Check sheet for the modelled part. Datum: model origin and axes. Units: mm. A direction names the side the tool comes from. Coordinates: 2 decimals unless noted, no trailing zeros. Order: outer loops, then holes, each group sorted by start corner. A loop starts at its lowest first (then second) coordinate and runs counter-clockwise, first axis right, second up. Notation, with made-up numbers: (52.5, -21) -> (101.5, -21) arc R24 cw to (101.5, -10) -> close; hole circle Ø1 at (-15, -3.75). An arc over 180 degrees is marked (long way). Put each result on its own line as item: value. Start each with the question number.
```python
from build123d import *

# Parameters (mm, degrees)
F0_W     = 309.716136
F0_H     = 25.80601
F1_DEPTH = 114.3
F2_T     = -2.54


with BuildPart() as f1:
    # F0 (on Right) → F1 (new body)
    with BuildSketch(Plane.YZ):
        Rectangle(F0_W, F0_H)
    extrude(amount=F1_DEPTH)

    # F2
    f2_openings = [f1.faces().sort_by_distance(p)[0] for p in [
        (57.15, -154.858068, 0),
        (57.15, 0, 12.903005),
        (114.3, 0, 0),
        (57.15, 154.858068, 0),
    ]]
    offset(amount=F2_T, openings=f2_openings)


solid = f1.part
```
1) Gauge pin test, flat ends, axial feed: pin 1 (2 mm diameter, centred on y = 106, z = 4.5, fed in from +X); pin 2 (3 mm diameter, centred on x = 15, y = -82.5, fed in from +Z). Record the tip position at first contact, or that the pin passes through.
2) Sectioned sample at A-A (y = -115.5). Record the boundary of the cut face in (x, z).
3) Scan lines: line 1 along X through (y, z) = (-29, 10); line 2 along Z through (x, y) = (103, -69). Record each from-to range of solid material in increasing order. Write a range as [from, to].
4) Access from +Z, -Z, +X, -X, +Y, -Y to the whole of each face (thin tool, end or side, straight path). Record for faces 1 (the flat face through (58, -2, -10.363)), 2 (the flat face through (44, 154.858, -11)).
5) Sectioned sample at C-C (x = 88.5). Record the boundary of the cut face in (y, z).
6) Sectioned sample at B-B (z = -7.25). Record the boundary of the cut face in (x, y), plus the area to 3 significant figures.
Entries:
1. pin 1: stops at x = 2.54
1. pin 2: stops at z = -10.36
2. outline: (0, -12.9) -> (114.3, -12.9) -> (114.3, -10.36) -> (2.54, -10.36) -> (2.54, 12.9) -> (0, 12.9) -> close
3. line 1: x = [0, 2.54]
3. line 2: z = [-12.9, -10.36]
4. face 1: +Z, +X, +Y, -Y
4. face 2: +Z, -Z, +X, -X, +Y
5. outline: (-154.86, -12.9) -> (154.86, -12.9) -> (154.86, -10.36) -> (-154.86, -10.36) -> close
6. outline: (0, -154.86) -> (2.54, -154.86) -> (2.54, 154.86) -> (0, 154.86) -> close
6. area: 787 mm2
